```python
from build123d import *

# Parameters (mm, degrees)
F0_W     = 419.1
F0_H     = 552.45
F0_R     = 3.96875
F1_DEPTH = 6.35


with BuildPart() as f1:
    # F0 (on Top) → F1 (new body)
    with BuildSketch(Plane.XY):
        with Locations((209.55, 276.225)):
            Rectangle(F0_W, F0_H)
        with Locations((9.454559, 9.666916)):
            Circle(F0_R, mode=Mode.SUBTRACT)
        with BuildLine():
            Line((133.35, 12.84139), (19.05, 12.84139))
            ThreePointArc((19.05, 12.84139), (14.559872, 14.701262), (12.7, 19.19139))
            Line((12.7, 19.19139), (12.7, 133.49139))
            ThreePointArc((12.7, 133.49139), (14.559872, 137.981518), (19.05, 139.84139))
            Line((19.05, 139.84139), (133.35, 139.84139))
            ThreePointArc((133.35, 139.84139), (137.840128, 137.981518), (139.7, 133.49139))
            Line((139.7, 133.49139), (139.7, 19.19139))
            ThreePointArc((139.7, 19.19139), (137.840128, 14.701262), (133.35, 12.84139))
        make_face(mode=Mode.SUBTRACT)
        with Locations((142.804305, 9.666916)):
            Circle(F0_R, mode=Mode.SUBTRACT)
        with BuildLine():
            Line((272.979305, 133.420695), (272.979305, 19.120695))
            ThreePointArc((272.979305, 19.120695), (271.119433, 14.630567), (266.629305, 12.770695))
            Line((266.629305, 12.770695), (152.329305, 12.770695))
            ThreePointArc((152.329305, 12.770695), (147.839177, 14.630567), (145.979305, 19.120695))
            Line((145.979305, 19.120695), (145.979305, 133.420695))
            ThreePointArc((145.979305, 133.420695), (147.839177, 137.910823), (152.329305, 139.770695))
            Line((152.329305, 139.770695), (266.629305, 139.770695))
            ThreePointArc((266.629305, 139.770695), (271.119433, 137.910823), (272.979305, 133.420695))
        make_face(mode=Mode.SUBTRACT)
        with Locations((9.454559, 142.945695)):
            Circle(F0_R, mode=Mode.SUBTRACT)
        with Locations((9.454559, 276.224473)):
            Circle(F0_R, mode=Mode.SUBTRACT)
        with BuildLine():
            Line((139.629305, 266.770695), (139.629305, 152.470695))
            ThreePointArc((139.629305, 152.470695), (137.769433, 147.980567), (133.279305, 146.120695))
            Line((133.279305, 146.120695), (18.979305, 146.120695))
            ThreePointArc((18.979305, 146.120695), (14.489177, 147.980567), (12.629305, 152.470695))
            Line((12.629305, 152.470695), (12.629305, 266.770695))
            ThreePointArc((12.629305, 266.770695), (14.489177, 271.260823), (18.979305, 273.120695))
            Line((18.979305, 273.120695), (133.279305, 273.120695))
            ThreePointArc((133.279305, 273.120695), (137.769433, 271.260823), (139.629305, 266.770695))
        make_face(mode=Mode.SUBTRACT)
        with Locations((142.804305, 142.945695)):
            Circle(F0_R, mode=Mode.SUBTRACT)
        with Locations((142.804305, 276.224473)):
            Circle(F0_R, mode=Mode.SUBTRACT)
        with Locations((276.154051, 9.666916)):
            Circle(F0_R, mode=Mode.SUBTRACT)
        with Locations((409.503797, 9.666916)):
            Circle(F0_R, mode=Mode.SUBTRACT)
        with BuildLine():
            Line((406.4, 133.35), (406.4, 19.05))
            ThreePointArc((406.4, 19.05), (404.540128, 14.559872), (400.05, 12.7))
            Line((400.05, 12.7), (285.75, 12.7))
            ThreePointArc((285.75, 12.7), (281.259872, 14.559872), (279.4, 19.05))
            Line((279.4, 19.05), (279.4, 133.35))
            ThreePointArc((279.4, 133.35), (281.259872, 137.840128), (285.75, 139.7))
            Line((285.75, 139.7), (400.05, 139.7))
            ThreePointArc((400.05, 139.7), (404.540128, 137.840128), (406.4, 133.35))
        make_face(mode=Mode.SUBTRACT)
        with Locations((276.154051, 142.945695)):
            Circle(F0_R, mode=Mode.SUBTRACT)
        with BuildLine():
            Line((273.05, 266.84139), (273.05, 152.54139))
            ThreePointArc((273.05, 152.54139), (271.190128, 148.051262), (266.7, 146.19139))
            Line((266.7, 146.19139), (152.4, 146.19139))
            ThreePointArc((152.4, 146.19139), (147.909872, 148.051262), (146.05, 152.54139))
            Line((146.05, 152.54139), (146.05, 266.84139))
            ThreePointArc((146.05, 266.84139), (147.909872, 271.331518), (152.4, 273.19139))
            Line((152.4, 273.19139), (266.7, 273.19139))
            ThreePointArc((266.7, 273.19139), (271.190128, 271.331518), (273.05, 266.84139))
        make_face(mode=Mode.SUBTRACT)
        with Locations((276.154051, 276.224473)):
            Circle(F0_R, mode=Mode.SUBTRACT)
        with Locations((409.503797, 142.945695)):
            Circle(F0_R, mode=Mode.SUBTRACT)
        with BuildLine():
            Line((406.4, 266.7), (406.4, 152.4))
            ThreePointArc((406.4, 152.4), (404.540128, 147.909872), (400.05, 146.05))
            Line((400.05, 146.05), (285.75, 146.05))
            ThreePointArc((285.75, 146.05), (281.259872, 147.909872), (279.4, 152.4))
            Line((279.4, 152.4), (279.4, 266.7))
            ThreePointArc((279.4, 266.7), (281.259872, 271.190128), (285.75, 273.05))
            Line((285.75, 273.05), (400.05, 273.05))
            ThreePointArc((400.05, 273.05), (404.540128, 271.190128), (406.4, 266.7))
        make_face(mode=Mode.SUBTRACT)
        with Locations((409.503797, 276.224473)):
            Circle(F0_R, mode=Mode.SUBTRACT)
        with BuildLine():
            Line((139.7, 400.05), (139.7, 285.75))
            ThreePointArc((139.7, 285.75), (137.840128, 281.259872), (133.35, 279.4))
            Line((133.35, 279.4), (19.05, 279.4))
            ThreePointArc((19.05, 279.4), (14.559872, 281.259872), (12.7, 285.75))
            Line((12.7, 285.75), (12.7, 400.05))
            ThreePointArc((12.7, 400.05), (14.559872, 404.540128), (19.05, 406.4))
            Line((19.05, 406.4), (133.35, 406.4))
            ThreePointArc((133.35, 406.4), (137.840128, 404.540128), (139.7, 400.05))
        make_face(mode=Mode.SUBTRACT)
        with Locations((9.454559, 409.503252)):
            Circle(F0_R, mode=Mode.SUBTRACT)
        with Locations((142.804305, 409.503252)):
            Circle(F0_R, mode=Mode.SUBTRACT)
        with BuildLine():
            Line((139.7, 533.4), (139.7, 419.1))
            ThreePointArc((139.7, 419.1), (137.840128, 414.609872), (133.35, 412.75))
            Line((133.35, 412.75), (19.05, 412.75))
            ThreePointArc((19.05, 412.75), (14.559872, 414.609872), (12.7, 419.1))
            Line((12.7, 419.1), (12.7, 533.4))
            ThreePointArc((12.7, 533.4), (14.559872, 537.890128), (19.05, 539.75))
            Line((19.05, 539.75), (133.35, 539.75))
            ThreePointArc((133.35, 539.75), (137.840128, 537.890128), (139.7, 533.4))
        make_face(mode=Mode.SUBTRACT)
        with Locations((9.454559, 542.78203)):
            Circle(F0_R, mode=Mode.SUBTRACT)
        with Locations((142.804305, 542.78203)):
            Circle(F0_R, mode=Mode.SUBTRACT)
        with BuildLine():
            Line((273.050001, 400.05), (273.050001, 285.75))
            ThreePointArc((273.050001, 285.75), (271.190129, 281.259872), (266.700001, 279.4))
            Line((266.700001, 279.4), (152.400001, 279.4))
            ThreePointArc((152.400001, 279.4), (147.909873, 281.259872), (146.050001, 285.75))
            Line((146.050001, 285.75), (146.050001, 400.05))
            ThreePointArc((146.050001, 400.05), (147.909873, 404.540128), (152.400001, 406.4))
            Line((152.400001, 406.4), (266.700001, 406.4))
            ThreePointArc((266.700001, 406.4), (271.190129, 404.540128), (273.050001, 400.05))
        make_face(mode=Mode.SUBTRACT)
        with Locations((276.154051, 409.503252)):
            Circle(F0_R, mode=Mode.SUBTRACT)
        with BuildLine():
            Line((406.4, 400.05), (406.4, 285.75))
            ThreePointArc((406.4, 285.75), (404.540128, 281.259872), (400.05, 279.4))
            Line((400.05, 279.4), (285.75, 279.4))
            ThreePointArc((285.75, 279.4), (281.259872, 281.259872), (279.4, 285.75))
            Line((279.4, 285.75), (279.4, 400.05))
            ThreePointArc((279.4, 400.05), (281.259872, 404.540128), (285.75, 406.4))
            Line((285.75, 406.4), (400.05, 406.4))
            ThreePointArc((400.05, 406.4), (404.540128, 404.540128), (406.4, 400.05))
        make_face(mode=Mode.SUBTRACT)
        with Locations((409.503797, 409.503252)):
            Circle(F0_R, mode=Mode.SUBTRACT)
        with BuildLine():
            Line((273.05, 533.4), (273.05, 419.1))
            ThreePointArc((273.05, 419.1), (271.190128, 414.609872), (266.7, 412.75))
            Line((266.7, 412.75), (152.4, 412.75))
            ThreePointArc((152.4, 412.75), (147.909872, 414.609872), (146.05, 419.1))
            Line((146.05, 419.1), (146.05, 533.4))
            ThreePointArc((146.05, 533.4), (147.909872, 537.890128), (152.4, 539.75))
            Line((152.4, 539.75), (266.7, 539.75))
            ThreePointArc((266.7, 539.75), (271.190128, 537.890128), (273.05, 533.4))
        make_face(mode=Mode.SUBTRACT)
        with Locations((276.154051, 542.78203)):
            Circle(F0_R, mode=Mode.SUBTRACT)
        with BuildLine():
            Line((406.4, 533.4), (406.4, 419.1))
            ThreePointArc((406.4, 419.1), (404.540128, 414.609872), (400.05, 412.75))
            Line((400.05, 412.75), (285.75, 412.75))
            ThreePointArc((285.75, 412.75), (281.259872, 414.609872), (279.4, 419.1))
            Line((279.4, 419.1), (279.4, 533.4))
            ThreePointArc((279.4, 533.4), (281.259872, 537.890128), (285.75, 539.75))
            Line((285.75, 539.75), (400.05, 539.75))
            ThreePointArc((400.05, 539.75), (404.540128, 537.890128), (406.4, 533.4))
        make_face(mode=Mode.SUBTRACT)
        with Locations((409.503797, 542.78203)):
            Circle(F0_R, mode=Mode.SUBTRACT)
    extrude(amount=F1_DEPTH)


solid = f1.part
```
Read the model definition and answer for the solid it produces. Units are mm, in the model's axes. Give positions to 0.01 mm unless a question says otherwise; leave off trailing zeros. Loops run counter-clockwise (first coordinate to the right, second up) from the corner with the lowest first, then second, coordinate; pieces in that order, holes last.
Item 1: Find the intervals of material crossed by line 1 along X through (y, z) = (441.5, 3); line 2 along Y through (x, z) = (96, 6.25); line 3 along Y through (x, z) = (196, 3), in increasing order.
Item 2: The part is cut by section C-C (z = 4.75). Give the number of separate pieces and of enclosed holes in the cut face, and give its area (3 significant figures).
Item 3: The part is cut by section A-A (y = 298). Write down the section's boundary in (x, z).
Item 4: The part is cut by section B-B (x = 124). Write down the section's boundary in (y, z).
Taken from the geometry:
1. line 1: x = 0 to 12.7, 139.7 to 146.05, 273.05 to 279.4, 406.4 to 419.1
1. line 2: y = 0 to 12.84, 139.84 to 146.12, 273.12 to 279.4, 406.4 to 412.75, 539.75 to 552.45
1. line 3: y = 0 to 12.77, 139.77 to 146.19, 273.19 to 279.4, 406.4 to 412.75, 539.75 to 552.45
2. separate pieces: 1
2. enclosed holes: 32
2. area: 37,400 mm2
3. outline: (0, 0) - (12.7, 0) - (12.7, 6.35) - (0, 6.35) - close; (139.7, 0) - (146.05, 0) - (146.05, 6.35) - (139.7, 6.35) - close; (273.05, 0) - (279.4, 0) - (279.4, 6.35) - (273.05, 6.35) - close; (406.4, 0) - (419.1, 0) - (419.1, 6.35) - (406.4, 6.35) - close
4. outline: (0, 0) - (12.84, 0) - (12.84, 6.35) - (0, 6.35) - close; (139.84, 0) - (146.12, 0) - (146.12, 6.35) - (139.84, 6.35) - close; (273.12, 0) - (279.4, 0) - (279.4, 6.35) - (273.12, 6.35) - close; (406.4, 0) - (412.75, 0) - (412.75, 6.35) - (406.4, 6.35) - close; (539.75, 0) - (552.45, 0) - (552.45, 6.35) - (539.75, 6.35) - close
